Build history of the part. All positions in model axes, mm. A direction names the side the tool comes from. Give positions to 0.01 mm unless a question says otherwise; leave off trailing zeros. Loops run counter-clockwise (first coordinate to the right, second up) from the corner with the lowest first, then second, coordinate; pieces in that order, holes last. Notation, with made-up numbers: (-24.5, 88.25) -> (17.5, 88.25) arc R36 cw to (17.5, 126.25) -> close; hole circle Ø11 at (80, 56.25). An arc over 180 degrees is marked (long way). Answer in a Markdown table with one row per item. Add a question column.
from build123d import *

# Parameters (mm, degrees)
EXTRUDE_1_DEPTH     = 60
SKETCH_2_R          = 11.75
CUT_EXTRUDE_1_DEPTH = 40
SKETCH_3_R          = 9.5
CUT_EXTRUDE_2_DEPTH = 40
M3X0_5_1_D          = 2.5
M3X0_5_1_DEPTH      = 5
M3X0_5_1_TIP        = 0.751075774
CUT_EXTRUDE_3_REACH = 18.2
SKETCH_7_R          = 1.65


with BuildPart() as part:
    # 草圖1 → 填料-伸長1 (new body)
    with BuildSketch(Plane.XY):
        Polygon((-25, 0), (-17, 0), (-17, 6), (17, 6), (17, 0), (25, 0), (25, 16.2), (-25, 16.2), align=None)
    extrude(amount=EXTRUDE_1_DEPTH)

    # 草圖2 → 除料-伸長1 (cut)
    with BuildSketch(Plane(origin=(0, 16.2, 0), x_dir=(1, 0, 0), z_dir=(0, 1, 0))):
        with Locations((0, -18.5)):
            Circle(SKETCH_2_R)
    extrude(amount=-CUT_EXTRUDE_1_DEPTH, mode=Mode.SUBTRACT)

    # 草圖3 → 除料-伸長2 (cut)
    with BuildSketch(Plane(origin=(0, 16.2, 0), x_dir=(1, 0, 0), z_dir=(0, 1, 0))):
        with Locations((0, -44.5)):
            Circle(SKETCH_3_R)
    extrude(amount=-CUT_EXTRUDE_2_DEPTH, mode=Mode.SUBTRACT)

    # M3x0.5 螺紋孔1
    with Locations(Plane(origin=(0, 16.2, 0), x_dir=(1, 0, 0), z_dir=(0, 1, 0))):
        with Locations((19, -44.5), (-19, -44.5)):
            Hole(M3X0_5_1_D / 2, depth=M3X0_5_1_DEPTH)
            with Locations((0, 0, -(M3X0_5_1_DEPTH + M3X0_5_1_TIP / 2))):  # 118° drill point
                Cone(0, M3X0_5_1_D / 2, M3X0_5_1_TIP, mode=Mode.SUBTRACT)

    # 草圖7 → 除料-伸長3 (cut, up to next)
    with BuildSketch(Plane(origin=(0, 16.2, 0), x_dir=(1, 0, 0), z_dir=(0, 1, 0)), mode=Mode.PRIVATE) as cut_extrude_3_sk1:
        with Locations((-21, -35)):
            Circle(SKETCH_7_R)
    cut_extrude_3_tool1 = extrude(cut_extrude_3_sk1.sketch, amount=-CUT_EXTRUDE_3_REACH, mode=Mode.PRIVATE) & part.part
    add(cut_extrude_3_tool1.solids().sort_by_distance((-21, 16.2, 35))[0], mode=Mode.SUBTRACT)
    # 草圖7 → 除料-伸長3 (cut, up to next)
    with BuildSketch(Plane(origin=(0, 16.2, 0), x_dir=(1, 0, 0), z_dir=(0, 1, 0)), mode=Mode.PRIVATE) as cut_extrude_3_sk2:
        with Locations((-21, -15)):
            Circle(SKETCH_7_R)
    cut_extrude_3_tool2 = extrude(cut_extrude_3_sk2.sketch, amount=-CUT_EXTRUDE_3_REACH, mode=Mode.PRIVATE) & part.part
    add(cut_extrude_3_tool2.solids().sort_by_distance((-21, 16.2, 15))[0], mode=Mode.SUBTRACT)
    # 草圖7 → 除料-伸長3 (cut, up to next)
    with BuildSketch(Plane(origin=(0, 16.2, 0), x_dir=(1, 0, 0), z_dir=(0, 1, 0)), mode=Mode.PRIVATE) as cut_extrude_3_sk3:
        with Locations((21, -35)):
            Circle(SKETCH_7_R)
    cut_extrude_3_tool3 = extrude(cut_extrude_3_sk3.sketch, amount=-CUT_EXTRUDE_3_REACH, mode=Mode.PRIVATE) & part.part
    add(cut_extrude_3_tool3.solids().sort_by_distance((21, 16.2, 35))[0], mode=Mode.SUBTRACT)
    # 草圖7 → 除料-伸長3 (cut, up to next)
    with BuildSketch(Plane(origin=(0, 16.2, 0), x_dir=(1, 0, 0), z_dir=(0, 1, 0)), mode=Mode.PRIVATE) as cut_extrude_3_sk4:
        with Locations((21, -15)):
            Circle(SKETCH_7_R)
    cut_extrude_3_tool4 = extrude(cut_extrude_3_sk4.sketch, amount=-CUT_EXTRUDE_3_REACH, mode=Mode.PRIVATE) & part.part
    add(cut_extrude_3_tool4.solids().sort_by_distance((21, 16.2, 15))[0], mode=Mode.SUBTRACT)


solid = part.part
(1) Flat gauge pins, fed straight in: pin 1 Ø5 at (x, z) = (-12, 28) entering from -Y; pin 2 Ø6 at (x, z) = (8.5, 18) entering from +Y; pin 3 Ø4.5 at (x, z) = (21, 15) entering from +Y. Where does each tip first touch, or does it go through?
(2) Saw through at A-A, the plane x = 21. List the corners of the cut face in (y, z), then the cut area to 3 significant figures.
(3) 3-axis set-ups, long thin cutter, end or side, ignore diameter. For faces 1 (the flat face through (-17, 3, 30)), 2 (the flat face through (-21, 0, 30)), 3 (the cylindrical face through (-19.672, 13.665, 43.446)): which of +Z, -Z, +X, -X, +Y, -Y reach the whole face in a straight line?
(4) Saw through at B-B, the plane y = 14. State how many separate pieces and enclosed holes the cut face has, then the cut area to 3 significant figures.
(5) Saw through at C-C, the plane z = 4. List the corners of the cut face in (x, y).
(6) Saw through at D-D, the plane z = 18.5. List the corners of the cut face in (x, y), then the cut area to 3 significant figures.
(7) Two-plate mould, pull along X, no slides. Class faces 4 (the flat face through (0, 10, 0)), 5 (the cylindrical face through (-1.53, 11.17, 6.85)), 6 (the flat face through (-25, 8, 30)): released by +X, released by -X, zero draft, split by the parting line, or undercut.
(8) Wall check: line 1 along Z through (x, y) = (21, 10.5); line 2 along X through (y, z) = (14.75, 44.5); line 3 along Z through (x, y) = (0, 13.5). Give the ranges that are in metal, low to high. Write a range as from..to.
Worked answers:
| question | item | result |
|---|---|---|
| 1 | pin 1 | y = 6 |
| 1 | pin 2 | through |
| 1 | pin 3 | y = 16.2 |
| 2 | outline | (0, 0) -> (16.2, 0) -> (16.2, 13.35) -> (0, 13.35) -> close; (0, 16.65) -> (16.2, 16.65) -> (16.2, 33.35) -> (0, 33.35) -> close; (0, 36.65) -> (16.2, 36.65) -> (16.2, 60) -> (0, 60) -> close |
| 2 | area | 865 mm^2 |
| 3 | face 1 | +Z, -Z, -Y |
| 3 | face 2 | +Z, -Z, +X, -X, -Y |
| 3 | face 3 | +Y |
| 4 | separate pieces | 1 |
| 4 | enclosed holes | 8 |
| 4 | area | 2,240 mm^2 |
| 5 | outline | (-25, 0) -> (-17, 0) -> (-17, 6) -> (17, 6) -> (17, 0) -> (25, 0) -> (25, 16.2) -> (-25, 16.2) -> close |
| 6 | outline | (-25, 0) -> (-17, 0) -> (-17, 6) -> (-11.75, 6) -> (-11.75, 16.2) -> (-25, 16.2) -> close; (11.75, 6) -> (17, 6) -> (17, 0) -> (25, 0) -> (25, 16.2) -> (11.75, 16.2) -> close |
| 6 | area | 366 mm^2 |
| 7 | face 4 | zero draft |
| 7 | face 5 | undercut |
| 7 | face 6 | released by -X |
| 8 | line 1 | 0..13.35, 16.65..33.35, 36.65..60 |
| 8 | line 2 | -25..-20.25, -17.75..-9.5, 9.5..17.75, 20.25..25 |
| 8 | line 3 | 0..6.75, 30.25..35, 54..60 |
